```python
from build123d import *

# Parameters (mm, degrees)
BOSS_EXTRUDE1_DEPTH = 2.1
BOSS_EXTRUDE2_START = -1.4
SKETCH2_R           = 2.5
BOSS_EXTRUDE2_DEPTH = 1.4
SKETCH3_W           = 11.5
SKETCH3_H           = 6
CUT_EXTRUDE1_DEPTH  = 22.823152843
CHAMFER1_SIZE       = 2.5
CHAMFER1_SIZE2      = 4


with BuildPart() as part:
    # Sketch1 → Boss-Extrude1 (new body)
    with BuildSketch(Plane(origin=(0, 0, 0), x_dir=(1, 0, 0), z_dir=(0, 1, 0))):
        with BuildLine():
            Line((-5.75, 2.5), (-2.5, 5.75))
            Line((-2.5, 5.75), (-0.75, 5.75))
            Line((-0.75, 5.75), (-0.75, 7.964766161))
            ThreePointArc((-0.75, 7.964766161), (-5.916079783, 5.385164807), (-8, 0))
            Line((-8, 0), (-8, -20))
            Line((-8, -20), (8, -20))
            Line((8, -20), (8, 0))
            ThreePointArc((8, 0), (5.916079783, 5.385164807), (0.75, 7.964766161))
            Line((0.75, 7.964766161), (0.75, 5.75))
            Line((0.75, 5.75), (2.5, 5.75))
            Line((2.5, 5.75), (5.75, 2.5))
            Line((5.75, 2.5), (5.75, -6.75))
            Line((5.75, -6.75), (-5.75, -6.75))
            Line((-5.75, -6.75), (-5.75, 2.5))
        make_face()
    extrude(amount=BOSS_EXTRUDE1_DEPTH)

    # Sketch2 → Boss-Extrude2 (add)
    with BuildSketch(Plane(origin=(0, 0, 0), x_dir=(1, 0, 0), z_dir=(0, 1, 0)).offset(BOSS_EXTRUDE2_START)):
        with BuildLine():
            Line((8, 0), (8, -20))
            Line((8, -20), (-8, -20))
            Line((-8, -20), (-8, 0))
            ThreePointArc((-8, 0), (0, 8), (8, 0))
        make_face()
        with Locations(Location((0, 0, 0), (0, 0, 270))):
            Circle(SKETCH2_R, mode=Mode.SUBTRACT)
        with BuildLine():
            Line((-5, -5.5), (-5, -6.75))
            Line((-5, -6.75), (-3.5, -6.75))
            Line((-3.5, -6.75), (-3.5, -5.5))
            ThreePointArc((-3.5, -5.5), (-4.25, -4.75), (-5, -5.5))
        make_face(mode=Mode.SUBTRACT)
        with BuildLine():
            Line((3.5, -5.5), (3.5, -6.75))
            Line((3.5, -6.75), (5, -6.75))
            Line((5, -6.75), (5, -5.5))
            ThreePointArc((5, -5.5), (4.25, -4.75), (3.5, -5.5))
        make_face(mode=Mode.SUBTRACT)
    extrude(amount=BOSS_EXTRUDE2_DEPTH)

    # Sketch3 → Cut-Extrude1 (cut, through all)
    with BuildSketch(Plane(origin=(0, 2.1, 0), x_dir=(1, 0, 0), z_dir=(0, 1, 0))):
        with Locations((0, -9.75)):
            Rectangle(SKETCH3_W, SKETCH3_H)
    extrude(amount=-CUT_EXTRUDE1_DEPTH, mode=Mode.SUBTRACT)

    # Chamfer1
    chamfer1_edges = [part.edges().sort_by_distance(p)[0] for p in [
        (0, -1.4, 12.75),
    ]]
    chamfer1_side = [part.faces().sort_by_distance(p)[0] for p in [
        (0, 0.35, 12.75),
    ]]
    chamfer(chamfer1_edges, length=CHAMFER1_SIZE, length2=CHAMFER1_SIZE2, reference=chamfer1_side[0])


solid = part.part
```
Part model, mm, in its own coordinate system. A direction names the side the tool comes from. Round coordinates to 2 decimals unless told otherwise and drop trailing zeros. Order: outer loops, then holes, each group sorted by start corner. A loop starts at its lowest first (then second) coordinate and runs counter-clockwise, first axis right, second up. Notation, with made-up numbers: M -27.5,-34 L -11.5,-34 A32 ccw -11.5,2 Z; hole C 81,29.5 d3. An arc over 180 degrees is marked long. Answer in a Markdown table with one row per item. Add a question column.
Q1. Mould opens along Z. For faces 4 (the face through (4.1, 1.04, -4.15)), 5 (the face through (-0.75, 1, -7)), 6 (the face through (-3.5, -1, 6)), 7 (the face through (0, 0, 20)) say: +Z half, -Z half, draft (parallel to the pull), parting line (faces both ways), or undercut.
Q2. Cut at B-B on x = 4.25. Give the cut face in (y, z).
Q3. Wall check: L1, parallel to X at y = -0.95, z = 0; L2, parallel to X at y = 0.5, z = 7.5; L3, parallel to Z at x = 2, y = -0.5. Give the ranges that are in metal, low to high. Write a range as from..to.
Q4. Pin check, flat tips, straight feed: pin 1 (4.5 mm diameter, centred on x = 0, z = 0, fed in from +Y); pin 2 (1 mm diameter, centred on y = 1.5, z = -6.5, fed in from -X); pin 3 (1.7 mm diameter, centred on y = 1, z = -6.5, fed in from +X); pin 4 (6 mm diameter, centred on x = 0, z = 2, fed in from +Y). Stop position of each tip, or through.
Q5. Cut at A-A on z = 7.5. Give the cut face in (x, y).
Q6. 3-axis set-ups, long thin cutter, end or side, ignore diameter. For faces 1 (the face through (-4.15, 1.04, -4.1)), 2 (the face through (-4.23, -0.71, 4.75)), 3 (the face through (0.75, 1, -7)): which of +Z, -Z, +X, -X, +Y, -Y reach the whole face in a straight line?
Q7. Cut at D-D on x = 6.5. Give the cut face in (y, z), and give its area (3 significant figures).
Q8. Cut at C-C on x = 1.5. Give the cut face in (y, z), and give its area (3 significant figures).
Established:
| question | item | result |
|---|---|---|
| 1 | face 4 | undercut |
| 1 | face 5 | draft |
| 1 | face 6 | undercut |
| 1 | face 7 | +Z half |
| 2 | outline | M -1.4,-6.78 L 2.1,-6.78 L 2.1,-4 L 0,-4 L 0,4.75 L -1.4,4.75 Z; M -1.4,16.75 L 1.1,12.75 L 2.1,12.75 L 2.1,20 L -1.4,20 Z |
| 3 | L1 | x = -8..-2.5, 2.5..8 |
| 3 | L2 | x = -8..-5.75, 5.75..8 |
| 3 | L3 | z = -7.75..-1.5, 1.5..6.75, 15.31..20 |
| 4 | pin 1 | passes through |
| 4 | pin 2 | stops at x = -5.29 |
| 4 | pin 3 | stops at x = 5.66 |
| 4 | pin 4 | stops at y = 0 |
| 5 | outline | M -8,-1.4 L -5.75,-1.4 L -5.75,2.1 L -8,2.1 Z; M 5.75,-1.4 L 8,-1.4 L 8,2.1 L 5.75,2.1 Z |
| 6 | face 1 | +Y |
| 6 | face 2 | +Y, -Y |
| 6 | face 3 | -Z, +Y |
| 7 | outline | M -1.4,-4.66 L 2.1,-4.66 L 2.1,20 L -1.4,20 Z |
| 7 | area | 86.3 mm2 |
| 8 | outline | M -1.4,-7.86 L 2.1,-7.86 L 2.1,-5.75 L 0,-5.75 L 0,-2 L -1.4,-2 Z; M -1.4,2 L 0,2 L 0,6.75 L -1.4,6.75 Z; M -1.4,16.75 L 1.1,12.75 L 2.1,12.75 L 2.1,20 L -1.4,20 Z |
| 8 | area | 39.7 mm2 |
